The model under review builds one solid part; all positions refer to its coordinate system, in mm. A direction names the side the tool comes from. Give positions to 0.01 mm unless a question says otherwise; leave off trailing zeros. Loops run counter-clockwise (first coordinate to the right, second up) from the corner with the lowest first, then second, coordinate; pieces in that order, holes last. Notation, with made-up numbers: M -2,62.25 L 28,62.25 A16 cw 28,83.25 Z; hole C 17.5,-9.75 d9. An arc over 180 degrees is marked long. Return JSON: item names as keys, results as strings.
```python
from build123d import *

# Parameters (mm, degrees)
SKETCH1_R           = 3.5
BOSS_EXTRUDE1_DEPTH = 4.5
SKETCH2_R           = 2.5
CUT_EXTRUDE1_DEPTH  = 1
SKETCH3_R           = 2.5
CUT_EXTRUDE2_DEPTH  = 3
SKETCH4_R           = 1.25
CUT_EXTRUDE3_DEPTH  = 4.5
BOSS_EXTRUDE2_DEPTH = 1.5
SKETCH6_R           = 0.5
CUT_EXTRUDE4_DEPTH  = 5.5


with BuildPart() as part:
    # Sketch1 → Boss-Extrude1 (new body)
    with BuildSketch(Plane(origin=(0, 0, 0), x_dir=(1, 0, 0), z_dir=(0, 1, 0))):
        Circle(SKETCH1_R)
    extrude(amount=BOSS_EXTRUDE1_DEPTH)

    # Sketch2 → Cut-Extrude1 (cut)
    with BuildSketch(Plane(origin=(0, 4.5, 0), x_dir=(1, 0, 0), z_dir=(0, 1, 0))):
        Circle(SKETCH2_R)
    extrude(amount=-CUT_EXTRUDE1_DEPTH, mode=Mode.SUBTRACT)

    # Sketch3 → Cut-Extrude2 (cut)
    with BuildSketch(Plane.XZ):
        Circle(SKETCH3_R)
    extrude(amount=-CUT_EXTRUDE2_DEPTH, mode=Mode.SUBTRACT)

    # Sketch4 → Cut-Extrude3 (cut, through all)
    with BuildSketch(Plane(origin=(0, 3.5, 0), x_dir=(1, 0, 0), z_dir=(0, 1, 0))):
        Circle(SKETCH4_R)
    extrude(amount=-CUT_EXTRUDE3_DEPTH, mode=Mode.SUBTRACT)

    # Sketch5 → Boss-Extrude2 (add)
    with BuildSketch(Plane(origin=(0, 4.5, 0), x_dir=(1, 0, 0), z_dir=(0, 1, 0))):
        with BuildLine():
            Line((2.165063509, 2.75), (14.125822824, 1.99603823))
            ThreePointArc((14.125822824, 1.99603823), (16, 0), (14.125822824, -1.99603823))
            Line((14.125822824, -1.99603823), (2.165063509, -2.75))
            ThreePointArc((2.165063509, -2.75), (3.5, 0), (2.165063509, 2.75))
        make_face()
    extrude(amount=-BOSS_EXTRUDE2_DEPTH)

    # Sketch6 → Cut-Extrude4 (cut, through all)
    with BuildSketch(Plane(origin=(0, 4.5, 0), x_dir=(1, 0, 0), z_dir=(0, 1, 0))):
        with Locations((4.5, 0)):
            Circle(SKETCH6_R)
        with Locations((6.5, 0)):
            Circle(SKETCH6_R)
        with Locations((8.5, 0)):
            Circle(SKETCH6_R)
        with Locations((10.5, 0)):
            Circle(SKETCH6_R)
        with Locations((12.5, 0)):
            Circle(SKETCH6_R)
        with Locations((14.5, 0)):
            Circle(SKETCH6_R)
    extrude(amount=-CUT_EXTRUDE4_DEPTH, mode=Mode.SUBTRACT)


solid = part.part
```
1) Consider section C-C on z = 0.75. Write out the cut boundary in (x, y).
From the geometry:
{"outline": "M -3.42,0 L -2.38,0 L -2.38,3 L -1,3 L -1,3.5 L -2.38,3.5 L -2.38,4.5 L -3.42,4.5 Z; M 1,3 L 2.38,3 L 2.38,0 L 3.42,0 L 3.42,3 L 15.85,3 L 15.85,4.5 L 2.38,4.5 L 2.38,3.5 L 1,3.5 Z"}
2) Consider section A-A on x = 0. Write out the cut boundary in (y, z).
From the geometry:
{"outline": "M 0,-3.5 L 4.5,-3.5 L 4.5,-2.5 L 3.5,-2.5 L 3.5,-1.25 L 3,-1.25 L 3,-2.5 L 0,-2.5 Z; M 0,2.5 L 3,2.5 L 3,1.25 L 3.5,1.25 L 3.5,2.5 L 4.5,2.5 L 4.5,3.5 L 0,3.5 Z"}
3) The part is to be moulded in two halves that separate along X. For faces 1 (the face through (-3.497, 2.218, -0.154)), 2 (the face through (9, 4, 0)), 3 (the face through (15, 4, 0)), 4 (the face through (6, 4.5, 1)), say which applies: released by +X, released by -X, zero draft, split by the parting line, or undercut.
From the geometry:
{"face 1": "split by the parting line", "face 2": "undercut", "face 3": "undercut", "face 4": "zero draft"}
4) Consider section B-B on y = 4.05. Write out the cut boundary in (x, z).
From the geometry:
{"outline": "M 2.17,-2.75 L 14.13,-2 A2 ccw 14.13,2 L 2.17,2.75 A3.5 ccw long Z; hole C 0,0 d5; hole C 4.5,0 d1; hole C 6.5,0 d1; hole C 8.5,0 d1; hole C 10.5,0 d1; hole C 12.5,0 d1; hole C 14.5,0 d1"}
5) Wall thickness on L1, parallel to Y at x = -1.5, z = -1; L2, parallel to Y at x = 11.5, z = -1.5; L3, parallel to Z at x = -2.25, y = 3.55: over which ranges is each line inside the solid? List them lowest first. Write a range as from..to.
From the geometry:
{"L1": "3..3.5", "L2": "3..4.5", "L3": "-2.68..-1.09, 1.09..2.68"}
6) Tool access review of faces 5 (the face through (2, 0, 2)), 6 (the face through (-0.54, 4.01, 2.44)), 7 (the face through (-1, 3, -1)): name each direction out of +Z, -Z, +X, -X, +Y, -Y from which nothing blocks a thin tool from reaching the whole face with its end or side.
From the geometry:
{"face 5": "+Z, -Z, +X, -X, -Y", "face 6": "+Y", "face 7": "-Y"}
7) Consider section D-D on y = 1.8. Write out the cut boundary in (x, z).
From the geometry:
{"outline": "C 0,0 d7; hole C 0,0 d5"}
8) Insertion check: pin 1 (4 mm diameter, centred on x = 0, z = 0, fed in from -Y); pin 2 (2 mm diameter, centred on y = 1.5, z = 0.5, fed in from +X); pin 3 (1.5 mm diameter, centred on y = 3, z = -1.5, fed in from +X); pin 4 (4 mm diameter, centred on x = 1, z = -0.5, fed in from -Y). Each pin has a flat end and moves straight along its axis. Give the tip position at first contact, or say it passes through.
From the geometry:
{"pin 1": "y = 3", "pin 2": "x = 3.5", "pin 3": "x = 15.85", "pin 4": "y = 0"}
